The listing builds one solid part. Answer for the finished solid, in the listing's coordinates (mm). Face numbers are marked on the shaded views. A direction names the side the tool comes from. Give positions to 0.01 mm unless a question says otherwise; leave off trailing zeros. Write each loop counter-clockwise with the first axis right and the second up, starting at its lowest first coordinate (ties: lowest second). Pieces come first, ordered by that corner, then holes. Notation, with made-up numbers: M 67,-26 L 125,-26 A21 ccw 125,11 Z; hole C 39.25,-15.5 d5. An arc over 180 degrees is marked long. Return JSON: item names as keys, results as strings.
from build123d import *

# Parameters (mm, degrees)
SKETCH1_W           = 14.142143214
SKETCH1_H           = 9.160251854
SKETCH1_R           = 1.25
BOSS_EXTRUDE1_DEPTH = 5.4
SKETCH2_R           = 2.5
CUT_EXTRUDE1_DEPTH  = 2.5


with BuildPart() as part:
    # Sketch1 → Boss-Extrude1 (new body)
    with BuildSketch(Plane.XY):
        Rectangle(SKETCH1_W, SKETCH1_H)
        with Locations(Location((0, 0, 0), (0, 0, 180))):
            Circle(SKETCH1_R, mode=Mode.SUBTRACT)
    extrude(amount=BOSS_EXTRUDE1_DEPTH)

    # Sketch2 → Cut-Extrude1 (cut)
    with BuildSketch(Plane.XY.offset(5.4)):
        Circle(SKETCH2_R)
    extrude(amount=-CUT_EXTRUDE1_DEPTH, mode=Mode.SUBTRACT)


solid = part.part
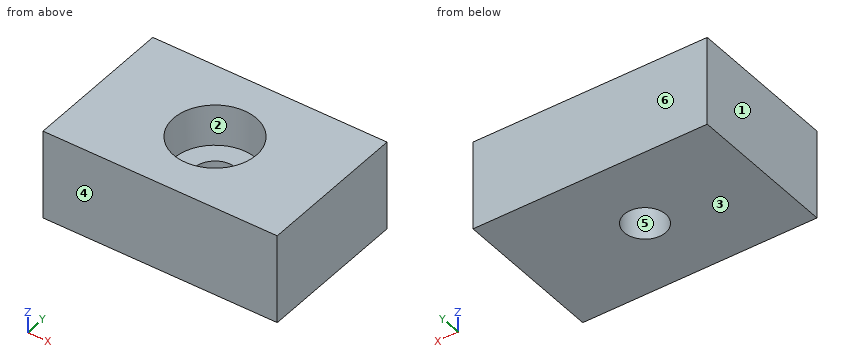
Item 1: Which of the six approach directions +Z, -Z, +X, -X, +Y, -Y give full straight-line access (tool end or side, diameter ignored) to the marked faces 1 and 2?
Geometry results:
{"face 1": "+Z, -Z, -X, +Y, -Y", "face 2": "+Z"}
Item 2: A cutting plane is placed at B-B, the plane x = 0. Write down the section's boundary in (y, z), plus the area to 3 significant figures.
Geometry results:
{"outline": "M -4.58,0 L -1.25,0 L -1.25,2.9 L -2.5,2.9 L -2.5,5.4 L -4.58,5.4 Z; M 1.25,0 L 4.58,0 L 4.58,5.4 L 2.5,5.4 L 2.5,2.9 L 1.25,2.9 Z", "area": "29.7 mm2"}
Item 3: A cutting plane is placed at A-A, the plane y = 0. Write down the section's boundary in (x, z), plus the area to 3 significant figures.
Geometry results:
{"outline": "M -7.07,0 L -1.25,0 L -1.25,2.9 L -2.5,2.9 L -2.5,5.4 L -7.07,5.4 Z; M 1.25,0 L 7.07,0 L 7.07,5.4 L 2.5,5.4 L 2.5,2.9 L 1.25,2.9 Z", "area": "56.6 mm2"}
Item 4: Given pin 1 Ø2 at (x, y) = (0, 0) entering from +Z, flat-ended and moving along its own axis, determine where the tip first touches the part or whether it passes through.
Geometry results:
{"pin 1": "passes through"}
Item 5: A cutting plane is placed at C-C, the plane z = 1.15. Write down the section's boundary in (x, y), plus the area to 3 significant figures.
Geometry results:
{"outline": "M -7.07,-4.58 L 7.07,-4.58 L 7.07,4.58 L -7.07,4.58 Z; hole C 0,0 d2.5", "area": "125 mm2"}
Item 6: Find the intervals of material crossed by line 1 (Y direction, x = 0, z = 4.1); line 2 (Z direction, x = 1.75, y = -0.75); line 3 (Y direction, x = 0, z = 1.15), in increasing order.
Geometry results:
{"line 1": "y = -4.58 to -2.5, 2.5 to 4.58", "line 2": "z = 0 to 2.9", "line 3": "y = -4.58 to -1.25, 1.25 to 4.58"}
Item 7: Determine the mould class of the marked faces 3, 4, 5 and 6 for opening direction Y: +Y half, -Y half, draft (parallel to the pull), parting line (faces both ways), or undercut.
Geometry results:
{"face 3": "draft", "face 4": "-Y half", "face 5": "undercut", "face 6": "+Y half"}
Item 8: A cutting plane is placed at D-D, the plane x = -1.5. Write down the section's boundary in (y, z).
Geometry results:
{"outline": "M -4.58,0 L 4.58,0 L 4.58,5.4 L 2,5.4 L 2,2.9 L -2,2.9 L -2,5.4 L -4.58,5.4 Z"}
